Part model, mm, in its own coordinate system. A direction names the side the tool comes from. Coordinates: 2 decimals unless noted, no trailing zeros. Order: outer loops, then holes, each group sorted by start corner. A loop starts at its lowest first (then second) coordinate and runs counter-clockwise, first axis right, second up.
from build123d import *

# Parameters (mm, degrees)
SKETCH004_W             = 218.2
SKETCH004_H             = 76.2
PAD004_DEPTH            = 1.75
SKETCH005_W             = 214.2
SKETCH005_H             = 72.2
PAD005_DEPTH            = 6.5
SKETCH006_W             = 184.2
SKETCH006_H             = 72.2
PAD006_DEPTH            = 12
BODY003_PLACEMENT_ANGLE = 180


with BuildPart() as part:
    # Sketch004 (on CopyDatumPlane) → Pad004 (new body)
    with BuildSketch(Plane(origin=(0, 0, -31.25), x_dir=(1, 0, 0), z_dir=(0, 0, -1))):
        Rectangle(SKETCH004_W, SKETCH004_H)
    extrude(amount=PAD004_DEPTH)

    # Sketch005 (on Face6 of Pad004) → Pad005 (join)
    with BuildSketch(Plane(origin=(0, 0, -33), x_dir=(1, 0, 0), z_dir=(0, 0, -1))):
        Rectangle(SKETCH005_W, SKETCH005_H)
    extrude(amount=PAD005_DEPTH)

    # Sketch006 (on Face11 of Pad005) → Pad006 (join)
    with BuildSketch(Plane(origin=(0, 0, -39.5), x_dir=(1, 0, 0), z_dir=(0, 0, -1))):
        with Locations((-5, 0)):
            Rectangle(SKETCH006_W, SKETCH006_H)
    extrude(amount=PAD006_DEPTH)


with BuildPart() as part_1:
    # Body003 placement: moved
    add(part.part.rotate(Axis((0, 0, 0), (0, 0, 1)), BODY003_PLACEMENT_ANGLE))


solid = part_1.part
Q1. Cut at D-D on z = -36. Write the cut outline in (x, y), and give its area (3 significant figures).
Results list:
outline: (-107.1, -36.1) - (107.1, -36.1) - (107.1, 36.1) - (-107.1, 36.1) - close
area: 15,500 mm2
Q2. Cut at C-C on z = -44.25. Write the cut outline in (x, y), and give its area (3 significant figures).
Results list:
outline: (-87.1, -36.1) - (97.1, -36.1) - (97.1, 36.1) - (-87.1, 36.1) - close
area: 13,300 mm2
Q3. Cut at B-B on y = -25.5. Write the cut outline in (x, z).
Results list:
outline: (-109.1, -33) - (-107.1, -33) - (-107.1, -39.5) - (-87.1, -39.5) - (-87.1, -51.5) - (97.1, -51.5) - (97.1, -39.5) - (107.1, -39.5) - (107.1, -33) - (109.1, -33) - (109.1, -31.25) - (-109.1, -31.25) - close
Q4. Cut at A-A on x = 82. Write the cut outline in (y, z).
Results list:
outline: (-38.1, -33) - (-36.1, -33) - (-36.1, -51.5) - (36.1, -51.5) - (36.1, -33) - (38.1, -33) - (38.1, -31.25) - (-38.1, -31.25) - close
Q5. Pin check, flat tips, straight feed: pin 1 Ø10 at (x, z) = (42, -48.5) entering from -Y; pin 2 Ø9.5 at (y, z) = (4, -48.5) entering from -X; pin 3 Ø6 at (x, z) = (23, -42.5) entering from +Y. Stop position of each tip, or through.
Results list:
pin 1: stops at y = -36.1
pin 2: stops at x = -87.1
pin 3: stops at y = 36.1
Q6. Which spindle directions (+Z, -Z, +X, -X, +Y, -Y) get a long thin tool onto all of the face, cutting with end or side? Do faces 1 (the face through (-97, 1, -39.5)), 2 (the face through (1, 36.1, -42)), 3 (the face through (2, 1, -31.25)), 4 (the face through (97.1, -1, -45)), 5 (the face through (1, -36.1, -42)). Say none if no direction does.
Results list:
face 1: -Z, -X, +Y, -Y
face 2: -Z, +X, -X, +Y
face 3: +Z, +X, -X, +Y, -Y
face 4: -Z, +X, +Y, -Y
face 5: -Z, +X, -X, -Y
Q7. Wall check: line 1 along X through (y, z) = (34, -42); line 2 along X through (y, z) = (-21.5, -39); line 3 along Y through (x, z) = (-84.5, -40.25). Give the ranges that are in metal, low to high.
Results list:
line 1: x = -87.1 to 97.1
line 2: x = -107.1 to 107.1
line 3: y = -36.1 to 36.1
